Design review of the part built by this model. Coordinates are the model's own, in mm. Face numbers are marked on the shaded views. A direction names the side the tool comes from. Round coordinates to 2 decimals unless told otherwise and drop trailing zeros. Loops run counter-clockwise (first coordinate to the right, second up) from the corner with the lowest first, then second, coordinate; pieces in that order, holes last. Notation, with made-up numbers: (70.25, 71.25) - (87.25, 71.25) arc R23 ccw to (87.25, 95.25) - close; hole circle Ø1 at (62, 87.25). An arc over 180 degrees is marked (long way). Return JSON: item names as keys, results as strings. Group by question number.
(1) Clearance check with flat-ended pins moving along their axes: pin 1 (3 mm diameter, centred on x = 36, z = 105, fed in from +Y); pin 2 (12 mm diameter, centred on x = 32.5, y = 13.5, fed in from +Z); pin 3 (1.6 mm diameter, centred on x = 17, z = 1, fed in from +Y). State where each tip first meets the part, or that it passes through.
(2) We need section D-D, the plane z = 31. Write out the cut boundary in (x, y).
(3) We need section B-B, the plane y = 11. Write out the cut boundary in (x, z), and give its area (3 significant figures).
(4) Wall thickness on L1, parallel to Y at x = 31, z = 102.65; L2, parallel to Z at x = 47, y = 2.5; L3, parallel to Z at x = 41, y = 8.5: over which ranges is each line inside the solid? List them lowest first. Write a range as [from, to].
(5) The part is to be moulded in two halves that separate along Z. For the marked faces 1, 2 and 3, say which applies: pulls with the +Z half, pulls with the -Z half, needs draft (parallel to the pull), parting line crosses it, or undercut.
(6) We need section C-C, the plane y = 5. Write out the cut boundary in (x, z).
(7) For the marked faces 4 and 5, list the 3-axis set-ups (+Z, -Z, +X, -X, +Y, -Y) from which the entire face can be reached by the end or side of a thin tool; tool diameter is ignored.
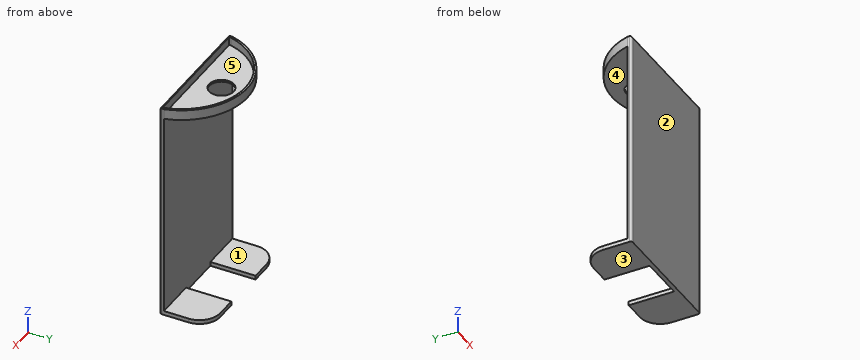
from build123d import *

# Parameters (mm, degrees)
BOSS_EXTRUDE1_DEPTH = 2
SKETCH4_W           = 62
SKETCH4_H           = 2
BOSS_EXTRUDE2_DEPTH = 100
BOSS_EXTRUDE3_DEPTH = 5
SHELL1_START        = 103
SHELL1_DEPTH        = 4
FILLET1_R           = 1
SKETCH7_R           = 6
CUT_EXTRUDE1_DEPTH  = 2
FILLET2_R           = 10
FILLET3_R           = 10


# Read off the part's stored shape, not the designer's step: Shell1
with BuildPart() as part:
    # Sketch3 → Boss-Extrude1 (new body)
    with BuildSketch(Plane.XY):
        Polygon((0, 0), (0, 24), (20, 24), (20, 2), (42, 2), (42, 24), (62, 24), (62, 0), align=None)
    extrude(amount=BOSS_EXTRUDE1_DEPTH)

    # Sketch4 → Boss-Extrude2 (add)
    with BuildSketch(Plane.XY.offset(2)):
        with Locations((31, 1)):
            Rectangle(SKETCH4_W, SKETCH4_H)
    extrude(amount=BOSS_EXTRUDE2_DEPTH)

    # Sketch6 → Boss-Extrude3 (add)
    with BuildSketch(Plane.XY.offset(102)):
        with BuildLine():
            Line((0, 2), (0, 0))
            Line((0, 0), (62, 0))
            Line((62, 0), (62, 2))
            ThreePointArc((62, 2), (31, 25.997977773), (0, 2))
        make_face()
    extrude(amount=BOSS_EXTRUDE3_DEPTH)

    # Shell1 outline → Shell1 (cut)
    with BuildSketch(Plane.XY.offset(SHELL1_START)):
        with BuildLine():
            Line((1, 1), (61, 1))
            Line((61, 1), (61, 1.871659386))
            ThreePointArc((61, 1.871659386), (31, 24.997977773), (1, 1.871659386))
            Line((1, 1.871659386), (1, 1))
        make_face()
    extrude(amount=SHELL1_DEPTH, mode=Mode.SUBTRACT)

    # Fillet1
    fillet1_edges = [part.edges().sort_by_distance(p)[0] for p in [
        (0, 0, 53.5),
        (62, 0, 53.5),
        (31, 0, 107),
    ]]
    fillet(fillet1_edges, radius=FILLET1_R - 0.0001)  # a hair under: the kernel refuses the full size

    # Sketch7 → Cut-Extrude1 (cut)
    with BuildSketch(Plane.XY.offset(103)):
        with Locations((31, 13.343458138)):
            Circle(SKETCH7_R)
    extrude(amount=-CUT_EXTRUDE1_DEPTH, mode=Mode.SUBTRACT)

    # Fillet2
    fillet2_edges = [part.edges().sort_by_distance(p)[0] for p in [
        (0, 24, 1),
    ]]
    fillet(fillet2_edges, radius=FILLET2_R)

    # Fillet3
    fillet3_edges = [part.edges().sort_by_distance(p)[0] for p in [
        (62, 24, 1),
    ]]
    fillet(fillet3_edges, radius=FILLET3_R)


solid = part.part
Solutions:
{
 "1": {"pin 1": "y = 25.81", "pin 2": "z = 103", "pin 3": "y = 24"},
 "2": {"outline": "(0, 1) arc R1 ccw to (1, 0) - (61, 0) arc R1 ccw to (62, 1) - (62, 2) - (0, 2) - close"},
 "3": {"outline": "(0, 0) - (20, 0) - (20, 2) - (0, 2) - close; (3.88, 102) - (25.48, 102) - (25.48, 103) - (5.07, 103) - (5.07, 107) - (3.88, 107) - close; (36.52, 102) - (58.12, 102) - (58.12, 107) - (56.93, 107) - (56.93, 103) - (36.52, 103) - close; (42, 0) - (62, 0) - (62, 2) - (42, 2) - close", "area": "133 mm^2"},
 "4": {"L1": "[0, 7.34], [19.34, 26]", "L2": "[0, 2], [102, 103]", "L3": "[102, 103]"},
 "5": {"face 1": "undercut", "face 2": "needs draft", "face 3": "pulls with the -Z half"},
 "6": {"outline": "(0, 0) - (20, 0) - (20, 2) - (0, 2) - close; (0.94, 102) - (61.06, 102) - (61.06, 107) - (60, 107) - (60, 103) - (2, 103) - (2, 107) - (0.94, 107) - close; (42, 0) - (62, 0) - (62, 2) - (42, 2) - close"},
 "7": {"face 4": "+X, -X, +Y", "face 5": "+Z"}
}
